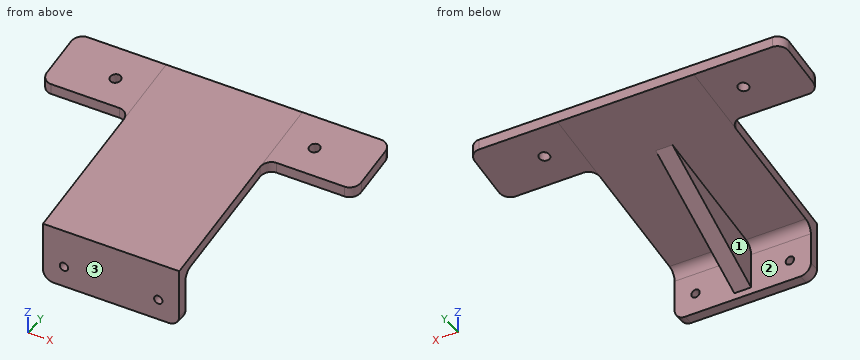
from build123d import *
from build123d.topology import SkipClean

# Parameters (mm, degrees)
BOSS_EXTRUDE1_DEPTH      = 65
SKETCH2_W                = 42.5
SKETCH2_H                = 30
BOSS_EXTRUDE2_DEPTH      = 5.000000239
FILLET1_R                = 5
CUT_EXTRUDE1_REACH       = 148.226
SKETCH3_R                = 2
SKETCH5_R                = 2.5
CUT_EXTRUDE2_DEPTH       = 149.107763403
BOSS_EXTRUDE3_DEPTH      = 4
BOSS_EXTRUDE3_DEPTH_BACK = 4


with BuildPart() as part:
    # Sketch1 → Boss-Extrude1 (new body)
    with BuildSketch(Plane(origin=(0, 0, 0), x_dir=(0, 0, -1), z_dir=(1, 0, 0))):
        Polygon((-17.632698071, 100), (0, 0), (28.3, 0), (28.3, 5), (4.118365096, 5), (-12.632698071, 100), align=None)
    extrude(amount=BOSS_EXTRUDE1_DEPTH)

    # Sketch2 → Boss-Extrude2 (add, along a direction that is not the sketch's normal)
    with SkipClean():  # the faces are left unmerged after this step: merging them gives an invalid solid
        with BuildSketch(Plane(origin=(0, 0, 0), x_dir=(1, 0, 0), z_dir=(0, -0.1736481776669274, 0.9848077530122086))):
            with Locations((-21.25, 86.542661189)):
                Rectangle(SKETCH2_W, SKETCH2_H)
            with Locations((86.25, 86.542661189)):
                Rectangle(SKETCH2_W, SKETCH2_H)
        extrude(amount=-BOSS_EXTRUDE2_DEPTH, dir=(0, 0, 1))

    # Fillet1
    fillet1_edges = [part.edges().sort_by_distance(p)[0] for p in [
        (32.5, 5, -4.118365096),
        (65, 2.5, -28.3),
        (0, 70.45576741, 9.923252622),
        (107.5, 70.45576741, 9.923252622),
        (65, 70.45576741, 9.923252622),
        (-42.5, 70.45576741, 9.923252622),
        (-42.5, 100, 15.132697952),
        (107.5, 100, 15.132697952),
        (0, 2.5, -28.3),
    ]]
    fillet(fillet1_edges, radius=FILLET1_R)

    # Sketch3 → Cut-Extrude1 (cut, up to next)
    with BuildSketch(Plane(origin=(0, 5, 0), x_dir=(1, 0, 0), z_dir=(0, 1, 0)), mode=Mode.PRIVATE) as cut_extrude1_sk1:
        with Locations(Location((10, 18.313863252, 0), (0, 0, 270))):
            Circle(SKETCH3_R)
    cut_extrude1_tool1 = extrude(cut_extrude1_sk1.sketch, amount=-CUT_EXTRUDE1_REACH, mode=Mode.PRIVATE) & part.part
    # Sketch3 → Cut-Extrude1 (cut, up to next)
    with BuildSketch(Plane(origin=(0, 5, 0), x_dir=(1, 0, 0), z_dir=(0, 1, 0)), mode=Mode.PRIVATE) as cut_extrude1_sk2:
        with Locations(Location((55, 18.313863252, 0), (0, 0, 270))):
            Circle(SKETCH3_R)
    cut_extrude1_tool2 = extrude(cut_extrude1_sk2.sketch, amount=-CUT_EXTRUDE1_REACH, mode=Mode.PRIVATE) & part.part
    add(cut_extrude1_tool1.solids().sort_by_distance((10, 5, -18.313863))[0], mode=Mode.SUBTRACT)
    add(cut_extrude1_tool2.solids().sort_by_distance((55, 5, -18.313863))[0], mode=Mode.SUBTRACT)

    # Sketch5 → Cut-Extrude2 (cut, through all)
    with SkipClean():  # the faces are left unmerged after this step: merging them gives an invalid solid
        with BuildSketch(Plane(origin=(0, 0.855050358, -4.849231552), x_dir=(-1, 0, 0), z_dir=(0, 0.1736481776669273, -0.9848077530122086))):
            with Locations(Location((-80, 85.6744203, 0), (0, 0, 90))):
                Circle(SKETCH5_R)
            with Locations(Location((15, 85.6744203, 0), (0, 0, 90))):
                Circle(SKETCH5_R)
        extrude(amount=-CUT_EXTRUDE2_DEPTH, mode=Mode.SUBTRACT)

    # Sketch9 → Boss-Extrude3 (add, two sides)
    with SkipClean():  # the faces are left unmerged after this step: merging them gives an invalid solid
        with BuildSketch(Plane.ZY.offset(-32.5)) as boss_extrude3_sk:
            with BuildLine():
                Line((-25.100344966, 5), (-8.313863252, 5))
                ThreePointArc((-8.313863252, 5), (-5.099925204, 6.169777784), (-3.389824487, 9.131759112))
                Line((-3.389824487, 9.131759112), (7.130723416, 68.796751166))
                Line((7.130723416, 68.796751166), (-25.100344966, 5))
            make_face()
        extrude(amount=BOSS_EXTRUDE3_DEPTH)
        extrude(boss_extrude3_sk.sketch, amount=-BOSS_EXTRUDE3_DEPTH_BACK)


solid = part.part
Work out the finished part from the listing and answer in its coordinate system (mm). Face numbers are marked on the shaded views. A direction names the side the tool comes from. Give positions to 0.01 mm unless a question says otherwise; leave off trailing zeros. Loops run counter-clockwise (first coordinate to the right, second up) from the corner with the lowest first, then second, coordinate; pieces in that order, holes last. Notation, with made-up numbers: (51.25, -2.75) -> (74.25, -2.75) arc R9 cw to (74.25, 7.25) -> close; hole circle Ø9 at (1, -8.5). An arc over 180 degrees is marked (long way). Use a Markdown table: item, result. Add a question column.
1. Section D-D on y = 57 is taken. Determine the outline of the cut face in (x, z).
2. Section B-B on y = 16 is taken. Determine the outline of the cut face in (x, z).
3. For the marked faces 1, 2 and 3, determine the directions among +Z, -Z, +X, -X, +Y, -Y from which every point of the face is accessible in a straight line to the end or side of a thin tool.
4. Find the intervals of material crossed by probe 1 along Y at (x, z) = (52.5, -9); probe 2 along X at (y, z) = (58.5, 7); probe 3 along X at (y, z) = (37.5, -5.5), in increasing order.
5. Flat-ended cylindrical pins translate along their axes: pin 1 Ø4 at (x, z) = (-14.5, 10) entering from -Y; pin 2 Ø9.5 at (y, z) = (29, -14.5) entering from -X; pin 3 Ø8 at (x, y) = (29, 78.5) entering from -Z. Find the tip coordinate at first contact, or state that the pin passes through.
6. Section A-A on x = 55 is taken. Determine the outline of the cut face in (y, z), and give its area (3 significant figures).
7. Section C-C on x = 84.5 is taken. Determine the outline of the cut face in (y, z).
Results below:
| question | item | result |
|---|---|---|
| 1 | outline | (0, 5.05) -> (28.5, 5.05) -> (28.5, 1.17) -> (36.5, 1.17) -> (36.5, 5.05) -> (65, 5.05) -> (65, 10.05) -> (0, 10.05) -> close |
| 2 | outline | (0, -2.18) -> (28.5, -2.18) -> (28.5, -19.54) -> (36.5, -19.54) -> (36.5, -2.18) -> (65, -2.18) -> (65, 2.82) -> (0, 2.82) -> close |
| 3 | face 1 | -Z, -X, +Y |
| 3 | face 2 | -Z, +Y |
| 3 | face 3 | +Z, -Z, +X, -X, -Y |
| 4 | probe 1 | y = 0 to 5 |
| 4 | probe 2 | x = 0 to 65 |
| 4 | probe 3 | x = 28.5 to 36.5 |
| 5 | pin 1 | stops at y = 70.46 |
| 5 | pin 2 | stops at x = 28.5 |
| 5 | pin 3 | stops at z = 8.14 |
| 6 | outline | (0, -28.3) -> (5, -28.3) -> (5, -20.31) -> (0, -20.31) -> close; (0, -16.31) -> (5, -16.31) -> (5, -8.31) arc R5 cw to (9.13, -3.39) -> (100, 12.63) -> (100, 17.63) -> (0, 0) -> close |
| 6 | area | 602 mm^2 |
| 7 | outline | (70.46, 7.42) -> (100, 12.63) -> (100, 17.63) -> (70.46, 12.42) -> close |
